Source: three-view drawing plus pictorial views. Frame: mm from the lowest corner of the part. Coordinates: 2 decimals unless noted, no trailing zeros. Order: outer loops, then holes, each group sorted by start corner. A loop starts at its lowest first (then second) coordinate and runs counter-clockwise, first axis right, second up. Notation, with made-up numbers: (-28.75, 7) - (-12.75, 7) arc R9 ccw to (-12.75, 23) - close; hole circle Ø6 at (89.5, 66.25). An arc over 180 degrees is marked (long way). One line per question, with ' | ' between items.
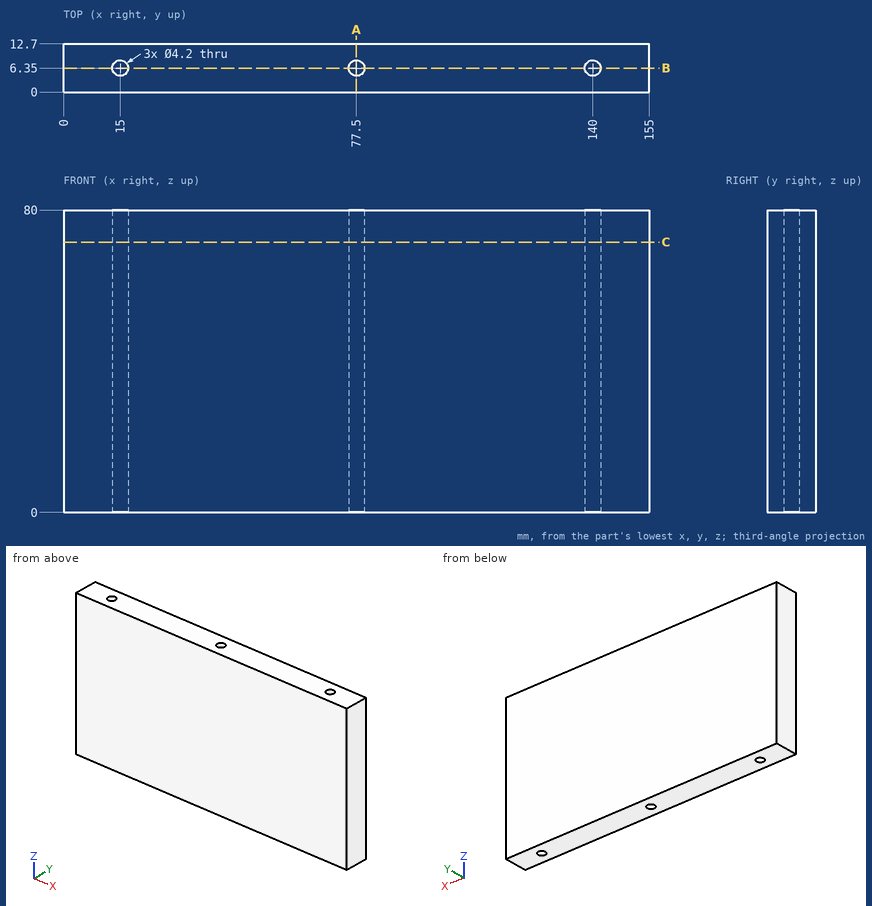
(1) Cut plane C-C (z = 71.5). Return the cut outline in (x, y).
Taken from the geometry:
outline: (0, 0) - (155, 0) - (155, 12.7) - (0, 12.7) - close; hole circle Ø4.2 at (15, 6.35); hole circle Ø4.2 at (77.5, 6.35); hole circle Ø4.2 at (140, 6.35)
(2) Cut plane B-B (y = 6.35). Return the cut outline in (x, z), and give its area (3 significant figures).
Taken from the geometry:
outline: (0, 0) - (12.9, 0) - (12.9, 80) - (0, 80) - close; (17.1, 0) - (75.4, 0) - (75.4, 80) - (17.1, 80) - close; (79.6, 0) - (137.9, 0) - (137.9, 80) - (79.6, 80) - close; (142.1, 0) - (155, 0) - (155, 80) - (142.1, 80) - close | area: 11,400 mm²
(3) Cut plane A-A (x = 77.5). Return the cut outline in (y, z).
Taken from the geometry:
outline: (0, 0) - (4.25, 0) - (4.25, 80) - (0, 80) - close; (8.45, 0) - (12.7, 0) - (12.7, 80) - (8.45, 80) - close
(4) Material intervals for L1, parallel to X at y = 6.5, z = 39; L2, parallel to Y at x = 77.5, z = 64; L3, parallel to Y at x = 76.5, z = 35, sorted ascending. Write a range as from..to.
Taken from the geometry:
L1: x = 0..12.91, 17.09..75.41, 79.59..137.91, 142.09..155 | L2: y = 0..4.25, 8.45..12.7 | L3: y = 0..4.5, 8.2..12.7
